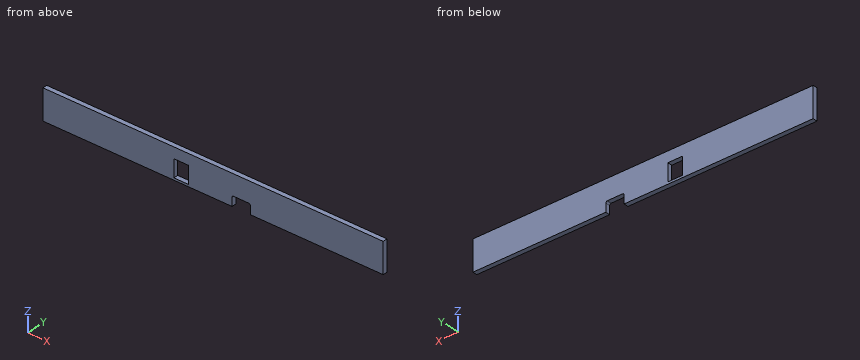
from build123d import *

# Parameters (mm, degrees)
SKETCH021_W     = 223
SKETCH021_H     = 3
PAD022_DEPTH    = 20
SKETCH022_W     = 9.5
SKETCH022_H     = 11.5
POCKET_DEPTH    = 3.001
POCKET001_DEPTH = 3.001


with BuildPart() as part:
    # Sketch021 → Pad022 (new body)
    with BuildSketch(Plane.XY):
        with Locations((0, -44.689828)):
            Rectangle(SKETCH021_W, SKETCH021_H)
    extrude(amount=PAD022_DEPTH)

    # Sketch022 (on Face3 of Pad022) → Pocket (cut, through all)
    with BuildSketch(Plane(origin=(0, -43.189828, 0), x_dir=(-1, 0, 0), z_dir=(0, 1, 0))):
        with Locations((20.955, 7.15)):
            Rectangle(SKETCH022_W, SKETCH022_H)
    extrude(amount=-POCKET_DEPTH, mode=Mode.SUBTRACT)

    # Sketch023 (on Face10 of Pocket) → Pocket001 (cut, through all)
    with BuildSketch(Plane(origin=(0, -43.189828, 0), x_dir=(-1, 0, 0), z_dir=(0, 1, 0))):
        with BuildLine():
            Line((-23.415, 6.5), (-13.415, 6.5))
            ThreePointArc((-12.415, 5.5), (-12.707893, 6.207107), (-13.415, 6.5))
            Line((-12.415, 5.5), (-12.415, -0.5))
            ThreePointArc((-13.415, -1.5), (-12.707893, -1.207107), (-12.415, -0.5))
            Line((-13.415, -1.5), (-23.415, -1.5))
            ThreePointArc((-24.415, -0.5), (-24.122107, -1.207107), (-23.415, -1.5))
            Line((-24.415, -0.5), (-24.415, 5.5))
            ThreePointArc((-23.415, 6.5), (-24.122107, 6.207107), (-24.415, 5.5))
        make_face()
    extrude(amount=-POCKET001_DEPTH, mode=Mode.SUBTRACT)


with BuildPart() as part_1:
    # Body013 placement: moved
    add(part.part.moved(Location((0, 88.392, 0))))


solid = part_1.part
Build history of the part. All positions in model axes, mm. Round coordinates to 2 decimals unless told otherwise and drop trailing zeros. Write each loop counter-clockwise with the first axis right and the second up, starting at its lowest first coordinate (ties: lowest second). Pieces come first, ordered by that corner, then holes. Notation, with made-up numbers: M -1,74.5 L 39,74.5 A24 cw 39,98.5 Z; hole C -37.75,78.5 d5. An arc over 180 degrees is marked long. Answer as a JSON object with one key per item and string values. Group by question number.
(1) Cut at A-A (z = 9). Give the cut face in (x, y) (3 decimals), and give its area (4 significant figures).
(2) Drill centre lines: L1, parallel to X at y = 42.4, z = 2.5 (3 decimals); L2, parallel to X at y = 44.9, z = 8.25 (3 decimals); L3, parallel to X at y = 43.1, z = 6.25 (3 decimals). Where is each one in solid material? Low to high.
(3) Cut at B-B (y = 44.6). Give the cut face in (x, z) (3 decimals), and give its area (3 significant figures).
(4) Flat gauge pin, fed straight in: pin 1 (1 mm diameter, centred on x = -11, y = 43, fed in from -Z). Where does the tip first touch, or does it go through?
Responses:
{
 "1": {"outline": "M -111.5,42.202 L -25.705,42.202 L -25.705,45.202 L -111.5,45.202 Z; M -16.205,42.202 L 111.5,42.202 L 111.5,45.202 L -16.205,45.202 Z", "area": "640.5 mm2"},
 "2": {"L1": "x = -111.5 to -25.705, -16.205 to 12.415, 24.415 to 111.5", "L2": "x = -111.5 to -25.705, -16.205 to 111.5", "L3": "x = -111.5 to -25.705, -16.205 to 12.754, 24.076 to 111.5"},
 "3": {"outline": "M -111.5,0 L 12.415,0 L 12.415,5.5 A1 cw 13.415,6.5 L 23.415,6.5 A1 cw 24.415,5.5 L 24.415,0 L 111.5,0 L 111.5,20 L -111.5,20 Z; hole M -25.705,1.4 L -16.205,1.4 L -16.205,12.9 L -25.705,12.9 Z", "area": "4,270 mm2"},
 "4": {"pin 1": "stops at z = 0"}
}
